Job drawing, mm, ordinate dimensions from the low corner. One solid piece. Coordinates: 2 decimals unless noted, no trailing zeros. Write each loop counter-clockwise with the first axis right and the second up, starting at its lowest first coordinate (ties: lowest second). Pieces come first, ordered by that corner, then holes. Notation, with made-up numbers: (-8.5, -6.5) -> (8.5, -6.5) arc R22 ccw to (8.5, 15.5) -> close; hole circle Ø7 at (-2.5, -19). An arc over 180 degrees is marked (long way). One line per question, with ' | ' between items. Start each with the question number.
Item 1: Saw through at A-A (y = 14.65). List the corners of the cut face in (x, z).
Item 2: Two-plate mould, pull along Y, no slides. Class the marked faces 1, 2 and 3: pulls with the +Y half, pulls with the -Y half, needs draft (parallel to the pull), parting line crosses it, or undercut.
Item 3: Pin check, flat tips, straight feed: pin 1 (3 mm diameter, centred on y = 9.5, z = 4, fed in from -X); pin 2 (2 mm diameter, centred on y = 17.5, z = 3, fed in from -X); pin 3 (10 mm diameter, centred on x = 14.65, y = 14.65, fed in from +Z). Stop position of each tip, or through.
Item 4: Probe probe 1 along Y at (x, z) = (14.65, 0.6); probe 2 along Y at (x, z) = (17, 3.95); probe 3 along Y at (x, z) = (3, 1.75). List the from-to ranges inside material, lowest first. Write a range as [from, to].
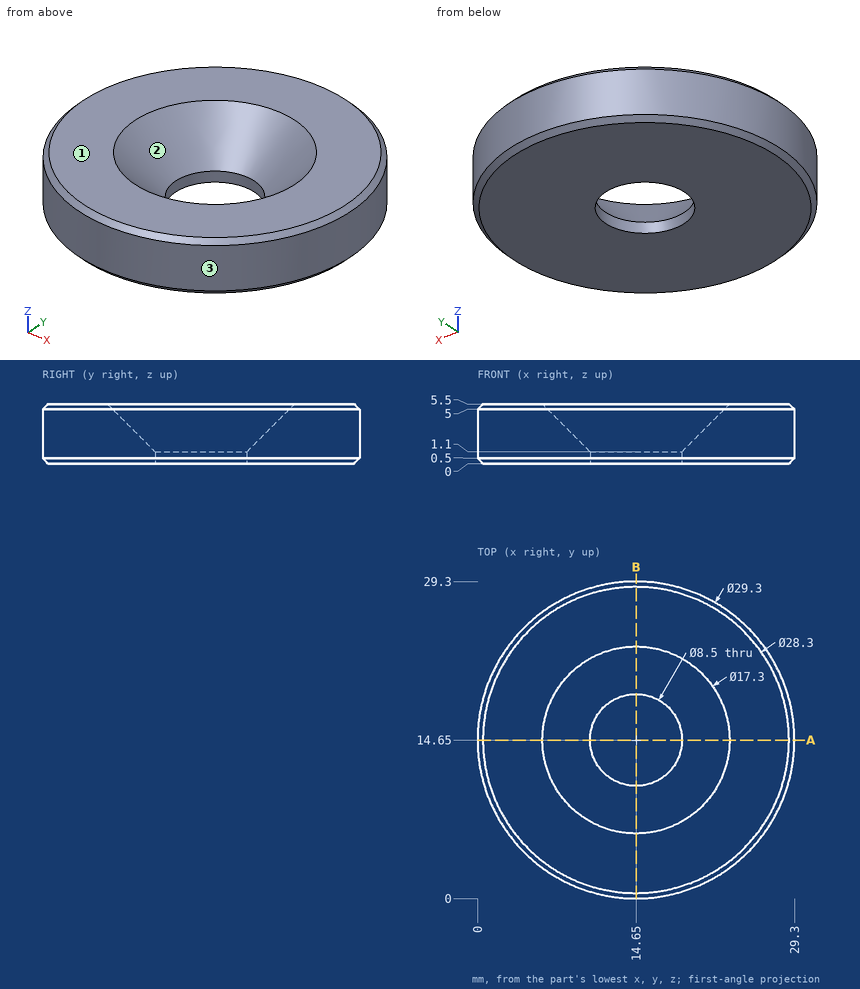
From the geometry:
1) outline: (0, 0.5) -> (0.5, 0) -> (10.4, 0) -> (10.4, 1.1) -> (6, 5.5) -> (0.5, 5.5) -> (0, 5) -> close; (18.9, 0) -> (28.8, 0) -> (29.3, 0.5) -> (29.3, 5) -> (28.8, 5.5) -> (23.3, 5.5) -> (18.9, 1.1) -> close
2) face 1: needs draft | face 2: undercut | face 3: parting line crosses it
3) pin 1: x = 0.46 | pin 2: x = 0.12 | pin 3: z = 1.85
4) probe 1: [0, 10.4], [18.9, 29.3] | probe 2: [0.19, 7.95], [21.35, 29.11] | probe 3: [5.77, 23.53]
